Build history of the part. All positions in model axes, mm. Round coordinates to 2 decimals unless told otherwise and drop trailing zeros. Write each loop counter-clockwise with the first axis right and the second up, starting at its lowest first coordinate (ties: lowest second). Pieces come first, ordered by that corner, then holes.
Autodesk Inventor part; units mm, degrees
ref_plane "YZ Plane" through (0, 0, 0) normal (1, 0, 0) x (0, 1, 0)
ref_plane "XZ Plane" through (0, 0, 0) normal (0, 1, 0) x (-1, 0, 0)
ref_plane "XY Plane" through (0, 0, 0) normal (0, 0, 1) x (1, 0, 0)
sketch "Sketch1" plane through (0, 0, 0) normal (0, 1, 0) x (-1, 0, 0)
  line L0 (0, 0) -> (130, 0)
  line L1 (130, 0) -> (130, -140)
  line L2 (130, -140) -> (0, -140)
  line L3 (0, -140) -> (0, 0)
  circle A0 centre (0, 0) radius 1.5
  circle A1 centre (130, 0) radius 1.5
  circle A2 centre (130, -140) radius 1.5
  circle A3 centre (0, -140) radius 1.5
  circle A4 centre (0, -140) radius 8
  circle A5 centre (130, -140) radius 8
  circle A6 centre (130, 0) radius 8
  circle A7 centre (0, 0) radius 8
  line L4 (130, 0) -> (0, 0) construction
  line L5 (130, -8) -> (0, -8)
  line L6 (0, 8) -> (130, 8)
  arc A8 (130, -8) -> (130, 8) centre (130, 0) ccw
  arc A9 (0, 8) -> (0, -8) centre (0, 0) ccw
  line L7 (130, -140) -> (0, -140) construction
  line L8 (130, -148) -> (0, -148)
  line L9 (0, -132) -> (130, -132)
  arc A10 (130, -148) -> (130, -132) centre (130, -140) ccw
  arc A11 (0, -132) -> (0, -148) centre (0, -140) ccw
  line L10 (65, 0) -> (65, -70)
  line L11 (65, -140) -> (65, 0) construction
  line L12 (73, -140) -> (73, 0)
  line L13 (57, 0) -> (57, -140)
  arc A12 (57, -140) -> (73, -140) centre (65, -140) ccw
  arc A13 (73, 0) -> (57, 0) centre (65, 0) ccw
  dimension "d0" = 130
  dimension "d1" = 140
  dimension "d2" = 3
  dimension "d3" = 3
  dimension "d4" = 3
  dimension "d5" = 3
  dimension "d6" = 16
  dimension "d7" = 16
  dimension "d8" = 16
  dimension "d9" = 16
  dimension "d10" = 70
  dimension "d14" = 8
extrude "Extrusion1" add sketch "Sketch1" along normal blind 3 contours A0 L3 A7 L0 | L0 A7 L3 A0 | A7 L6 A13 L0 | L0 L13 L5 A7 | A13 L0 | L0 L10 L5 L13 | A4 L2 A3 L3 | L9 L13 L2 A4 | L3 A3 L2 A4 | L5 L12 L9 L13 | L0 L12 L5 L10 | L6 A6 L0 A13 | L2 A12 L8 A4 | L9 L12 L2 L13 | L0 A6 L5 L12 | A6 L1 A1 L0 | L2 A12 | A12 L2 A5 L8 | L9 A5 L2 L12 | L0 A1 L1 A6 | A5 L2 A2 L1 | L1 A2 L2 A5
fillet "Fillet1" radius 20 4 edges at (-57, 1.5, -132) (-73, 1.5, -132) (-57, 1.5, -8) (-73, 1.5, -8)
properties part number "Handle 2"
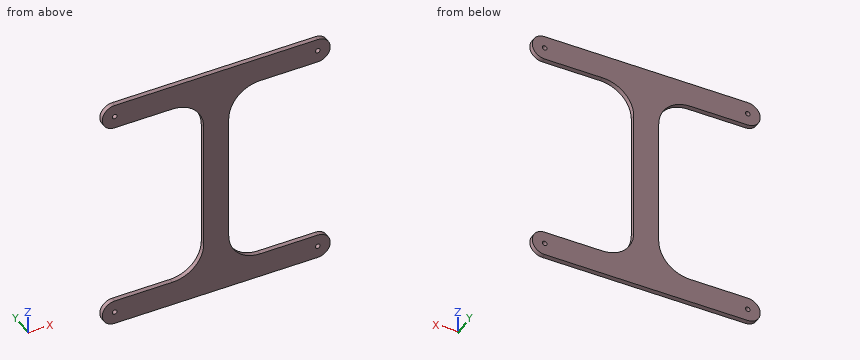
1) Slice it at B-B (y = 1.25). Write the cut outline in (x, z), plus the area to 3 significant figures.
Results:
outline: (-130, -148) - (0, -148) arc R8 ccw to (0, -132) - (-37, -132) arc R20 cw to (-57, -112) - (-57, -28) arc R20 cw to (-37, -8) - (0, -8) arc R8 ccw to (0, 8) - (-130, 8) arc R8 ccw to (-130, -8) - (-93, -8) arc R20 cw to (-73, -28) - (-73, -112) arc R20 cw to (-93, -132) - (-130, -132) arc R8 ccw to start; hole circle Ø3 at (-130, -140); hole circle Ø3 at (-130, 0); hole circle Ø3 at (0, -140); hole circle Ø3 at (0, 0)
area: 6,860 mm2
2) Wall check: L1, parallel to Z at x = -130, y = 1.25; L2, parallel to X at y = 1.2, z = -140; L3, parallel to Z at x = -124.5, y = 1.5. Give the ranges that are in metal, low to high.
Results:
L1: z = -148 to -141.5, -138.5 to -132, -8 to -1.5, 1.5 to 8
L2: x = -138 to -131.5, -128.5 to -1.5, 1.5 to 8
L3: z = -148 to -132, -8 to 8
3) Slice it at D-D (x = -86.5). Write the cut outline in (y, z), plus the area to 3 significant figures.
Results:
outline: (0, -148) - (3, -148) - (3, -130.91) - (0, -130.91) - close; (0, -9.09) - (3, -9.09) - (3, 8) - (0, 8) - close
area: 103 mm2
4) Slice it at A-A (x = -10). Write the cut outline in (y, z).
Results:
outline: (0, -148) - (3, -148) - (3, -132) - (0, -132) - close; (0, -8) - (3, -8) - (3, 8) - (0, 8) - close
5) Slice it at C-C (z = -78). Write the cut outline in (x, y).
Results:
outline: (-73, 0) - (-57, 0) - (-57, 3) - (-73, 3) - close
6) Pin check, flat tips, straight feed: pin 1 Ø5 at (x, z) = (-130, 0) entering from -Y; pin 2 Ø1.5 at (y, z) = (1.5, -56) entering from -X; pin 3 Ø1.5 at (y, z) = (1, -87.5) entering from +X. Stop position of each tip, or through.
Results:
pin 1: stops at y = 0
pin 2: stops at x = -73
pin 3: stops at x = -57
